Design review of the part built by this model. Coordinates are the model's own, in mm. A direction names the side the tool comes from. Round coordinates to 2 decimals unless told otherwise and drop trailing zeros. Order: outer loops, then holes, each group sorted by start corner. A loop starts at its lowest first (then second) coordinate and runs counter-clockwise, first axis right, second up.
from build123d import *

# Parameters (mm, degrees)
F0_R     = 23.5
F0_R_2   = 21.5
F1_DEPTH = 30
F2_W     = 47
F2_H     = 3
F3_DEPTH = 23.501
F4_W     = 2
F4_H     = 2
F5_ANGLE = 180


with BuildPart() as f1:
    # F0 (on Top) → F1 (new body)
    with BuildSketch(Plane.XY):
        Circle(F0_R)
        Circle(F0_R_2, mode=Mode.SUBTRACT)
    extrude(amount=F1_DEPTH)

    # F2 (on Right) → F3 (cut, through all)
    with BuildSketch(Plane.YZ):
        with Locations((0, 7.5)):
            Rectangle(F2_W, F2_H)
    extrude(amount=-F3_DEPTH, mode=Mode.SUBTRACT)

    # F4 (on Front) → F5 (revolve, symmetric)
    with BuildSketch(Plane.XZ) as f5_sk:
        with Locations((20.5, 10)):
            Rectangle(F4_W, F4_H)
        with Locations((20.5, 5)):
            Rectangle(F4_W, F4_H)
    revolve(axis=Axis((0, 0, 9.00836), (0, 0, 1)), revolution_arc=F5_ANGLE / 2)
    revolve(f5_sk.sketch, axis=Axis((0, 0, 9.00836), (0, 0, -1)), revolution_arc=F5_ANGLE / 2)


solid = f1.part
1) Take a section at B-B on x = 12. Give the boundary of the cut face in (y, z), plus the area to 3 significant figures.
Results:
outline: (-20.21, 0) - (-17.84, 0) - (-17.84, 4) - (-15.37, 4) - (-15.37, 6) - (-17.84, 6) - (-17.84, 9) - (-15.37, 9) - (-15.37, 11) - (-17.84, 11) - (-17.84, 30) - (-20.21, 30) - close; (15.37, 4) - (17.84, 4) - (17.84, 0) - (20.21, 0) - (20.21, 30) - (17.84, 30) - (17.84, 11) - (15.37, 11) - (15.37, 9) - (17.84, 9) - (17.84, 6) - (15.37, 6) - close
area: 162 mm2
2) The part is to be moulded in two halves that separate along Z. For faces 6 (the face through (0, 22, 8)), 7 (the face through (20, -2, 11)), 8 (the face through (10.33, -19.04, 0)), 9 (the face through (20, -2, 9)), say which applies: released by +Z, released by -Z, zero draft, split by the parting line, or undercut.
Results:
face 6: undercut
face 7: released by +Z
face 8: released by -Z
face 9: undercut
3) Take a section at D-D on z = 27.5. Give the boundary of the cut face in (x, y).
Results:
outline: circle Ø47 at (0, 0); hole circle Ø43 at (0, 0)
4) To check wall thickness, follow line 1 along Z through (x, y) = (20, -3); line 2 along X through (y, z) = (0, 3.75). State the ranges of each line that lie inside material, in increasing order.
Results:
line 1: z = 4 to 6, 9 to 11
line 2: x = -23.5 to -21.5, 21.5 to 23.5
5) For faces 1 (the face through (-21.48, 0.95, 19.35)), 2 (the face through (-21.48, 0.95, 2.29)), 3 (the face through (-22, 0, 6)), 4 (the face through (0, 20, 10)), 5 (the face through (21.495, -0.473, 7.479)), list the 3-axis set-ups (+Z, -Z, +X, -X, +Y, -Y) from which the entire face can be reached by the end or side of a thin tool; tool diameter is ignored.
Results:
face 1: +Z
face 2: -Z
face 3: -X, +Y, -Y
face 4: +Z, -Z
face 5: -X
6) Clearance check with flat-ended pins moving along their axes: P1, Ø6, axis at y = 9.5, z = 17, coming from the -X side; P2, Ø1, axis at y = 21, z = 5, coming from the -X side; P3, Ø1, axis at y = 20.5, z = 10, coming from the -X side. State where each tip first meets the part, or that it passes through.
Results:
P1: stops at x = -22.58
P2: stops at x = -11.49
P3: stops at x = -12.34
7) Take a section at C-C on x = -18. Give the boundary of the cut face in (y, z), plus the area to 3 significant figures.
Results:
outline: (-15.11, 0) - (-11.76, 0) - (-11.76, 6) - (-15.11, 6) - close; (-15.11, 9) - (-11.76, 9) - (-11.76, 30) - (-15.11, 30) - close; (11.76, 0) - (15.11, 0) - (15.11, 6) - (11.76, 6) - close; (11.76, 9) - (15.11, 9) - (15.11, 30) - (11.76, 30) - close
area: 181 mm2
8) Take a section at A-A on y = 0. Give the boundary of the cut face in (x, z), plus the area to 3 significant figures.
Results:
outline: (-23.5, 0) - (-21.5, 0) - (-21.5, 6) - (-23.5, 6) - close; (-23.5, 9) - (-21.5, 9) - (-21.5, 30) - (-23.5, 30) - close; (19.5, 4) - (21.5, 4) - (21.5, 0) - (23.5, 0) - (23.5, 30) - (21.5, 30) - (21.5, 11) - (19.5, 11) - (19.5, 9) - (21.5, 9) - (21.5, 6) - (19.5, 6) - close
area: 122 mm2
